For this review, take the finished solid that the model builds, in its own axes (mm). Face numbers are marked on the shaded views. Give positions to 0.01 mm unless a question says otherwise; leave off trailing zeros. Loops run counter-clockwise (first coordinate to the right, second up) from the corner with the lowest first, then second, coordinate; pieces in that order, holes last. Notation, with made-up numbers: (-17.5, 12) - (-2.5, 12) arc R11 ccw to (-2.5, 28) - close; hole circle Ø8 at (-3.75, -38). An arc over 180 degrees is marked (long way). Answer in a Markdown table with one row per item.
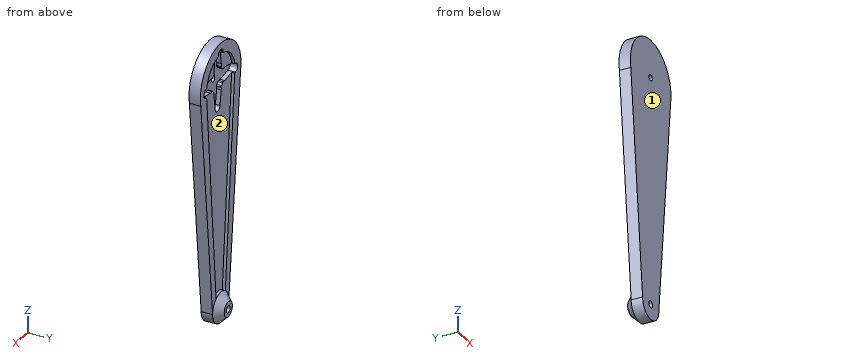
Autodesk Inventor part; units mm, degrees
ref_plane "Work Plane1" through (0, 12.5, 0) normal (0, 1, 0) x (1, 0, 0)
ref_plane "Work Plane2" through (0, 12.5, 0) normal (0, 1, 0) x (1, 0, 0)
ref_plane "YZ Plane" through (0, 0, 0) normal (1, 0, 0) x (0, 1, 0)
sketch "Sketch1" plane through (0, 0, 0) normal (0, 1, 0) x (-1, 0, 0)
  circle A0 centre (0, 0) radius 25
  line L0 (0, 0) -> (0, -150)
  circle A1 centre (0, -150) radius 10
  line L1 (0, 0) -> (25, 0)
  line L2 (0, -150) -> (10, -150)
  line L3 (0, -150) -> (-10, -150)
  line L4 (0, 0) -> (-25, 0)
  line L5 (25, 0) -> (10, -150)
  line L6 (-25, 0) -> (-10, -150)
  dimension "d0" = 50
  dimension "d1" = 150
  dimension "d2" = 20
extrude "Extrusion1" add sketch "Sketch1" along normal blind 7.5
sketch "Sketch2" plane through (0, 7.5, 0) normal (0, 1, 0) x (1, 0, 0)
  circle A0 centre (0, 0) radius 17.5
  arc A1 (10, 150) -> (-10, 150) centre (0, 150) ccw
  circle A2 centre (0, 150) radius 5
  line L0 (0, 0) -> (-17.5, 0)
  line L1 (0, 0) -> (17.5, 0)
  line L2 (0, 150) -> (-5, 150)
  line L3 (0, 150) -> (5, 150)
  line L4 (-17.5, 0) -> (-5, 150)
  line L5 (5, 150) -> (17.5, 0)
  dimension "d5" = 35
  dimension "d6" = 10
extrude "Extrusion2" cut sketch "Sketch2" against normal blind 2 contours L4 A0 L5 L1 L0 | L4 A2 L5 A0
sketch "Sketch3" plane through (0, 5.5, 0) normal (0, 1, 0) x (1, 0, 0)
  arc A0 (5, 150) -> (-5, 150) centre (0, 150) ccw
  circle A1 centre (0, 150) radius 2.25
  circle A2 centre (0, 0) radius 2
  dimension "d9" = 4.5
  dimension "d12" = 4
extrude "Extrusion4" cut sketch "Sketch3" against normal blind 5.5
sketch "Sketch4" plane through (0, 7.5, 0) normal (0, 1, 0) x (1, 0, 0)
  circle A0 centre (0, 150) radius 2.25
  arc A1 (5, 150) -> (-5, 150) centre (0, 150) ccw
  arc A2 (10, 150) -> (-10, 150) centre (0, 150) ccw
  line L0 (24.505, 4.9505) -> (10, 150)
  circle A3 centre (0, 150) radius 10
  circle A4 centre (0, 150) radius 2.25
  point P0 (0, 0)
  dimension "d22" = 4.5
ref_plane "Work Plane1" through (0, 12.5, 0) normal (0, 1, 0) x (1, 0, 0)
sketch "Sketch8" plane through (0, 5.5, 0) normal (0, 1, 0) x (1, 0, 0)
  point P0 (0, 0)
sketch "Sketch9" plane through (0, 7.5, 0) normal (0, 1, 0) x (1, 0, 0)
  arc A0 (2, 0) -> (-2, 0) centre (0, 0) ccw
  line L0 (17.5, 0) -> (-17.5, 0)
  circle A1 centre (0, 0) radius 17.5
extrude "Extrusion7" cut sketch "Sketch9" against normal blind 2 contours A0 L0 A1 | L0 A1
sketch "Sketch10" plane through (0, 7.5, 0) normal (0, 1, 0) x (1, 0, 0)
  arc A0 (-2.0881, -18.0545) -> (1.8643, -18.079) centre (-0.11, -17.7593) ccw
  line L0 (3.4056, -8.5599) -> (1.8643, -18.079)
  arc A1 (3.4056, -8.5599) -> (3.3448, -7.1465) centre (-0.0494, -8.0004) ccw
  arc A2 (4.0411, -5.092) -> (3.3448, -7.1465) centre (5.2844, -6.6585) ccw
  arc A3 (4.0411, -5.092) -> (5.0411, -4.1043) centre (0.0003, -0.0006) ccw
  arc A4 (7.1041, -3.4336) -> (5.0411, -4.1043) centre (6.5921, -5.367) ccw
  arc A5 (7.1041, -3.4336) -> (8.5166, -3.512) centre (8.0001, -0.0503) ccw
  line L1 (18.0541, -2.089) -> (8.5166, -3.512)
  arc A6 (18.0541, -2.089) -> (18.0787, 1.8634) centre (17.759, -0.1109) ccw
  line L2 (8.5596, 3.4047) -> (18.0787, 1.8634)
  arc A7 (8.5596, 3.4047) -> (7.1462, 3.344) centre (8.0001, -0.0503) ccw
  arc A8 (5.0917, 4.0402) -> (7.1462, 3.344) centre (6.6582, 5.2835) ccw
  arc A9 (5.0917, 4.0402) -> (4.104, 5.0402) centre (0.0003, -0.0006) ccw
  arc A10 (3.4333, 7.1032) -> (4.104, 5.0402) centre (5.3667, 6.5912) ccw
  arc A11 (3.4333, 7.1032) -> (3.5117, 8.5157) centre (0.05, 7.9993) ccw
  line L3 (2.0887, 18.0533) -> (3.5117, 8.5157)
  arc A12 (2.0887, 18.0533) -> (-1.8637, 18.0778) centre (0.1106, 17.7581) ccw
  line L4 (-3.405, 8.5587) -> (-1.8637, 18.0778)
  arc A13 (-3.405, 8.5587) -> (-3.3443, 7.1453) centre (0.05, 7.9993) ccw
  arc A14 (-4.0405, 5.0908) -> (-3.3443, 7.1453) centre (-5.2838, 6.6574) ccw
  arc A15 (-4.0405, 5.0908) -> (-5.0405, 4.1031) centre (0.0003, -0.0006) ccw
  arc A16 (-7.1035, 3.4325) -> (-5.0405, 4.1031) centre (-6.5915, 5.3658) ccw
  arc A17 (-7.1035, 3.4325) -> (-8.516, 3.5108) centre (-7.9996, 0.0491) ccw
  line L5 (-18.0536, 2.0878) -> (-8.516, 3.5108)
  arc A18 (-18.0536, 2.0878) -> (-18.0781, -1.8646) centre (-17.7585, 0.1097) ccw
  line L6 (-8.559, -3.4059) -> (-18.0781, -1.8646)
  arc A19 (-8.559, -3.4059) -> (-7.1456, -3.3451) centre (-7.9996, 0.0491) ccw
  arc A20 (-5.0911, -4.0414) -> (-7.1456, -3.3451) centre (-6.6577, -5.2847) ccw
  arc A21 (-5.0911, -4.0414) -> (-4.1034, -5.0414) centre (0.0003, -0.0006) ccw
  arc A22 (-3.4328, -7.1044) -> (-4.1034, -5.0414) centre (-5.3661, -6.5924) ccw
  arc A23 (-3.4328, -7.1044) -> (-3.5111, -8.5169) centre (-0.0494, -8.0004) ccw
  line L7 (-2.0881, -18.0545) -> (-3.5111, -8.5169)
  arc A24 (-18.2011, 3.0769) -> (-18.238, -2.8517) centre (-17.7585, 0.1097) ccw
  line L8 (-18.2011, 3.0769) -> (-8.6636, 4.4998)
  arc A25 (-6.8475, 4.3991) -> (-8.6636, 4.4998) centre (-7.9996, 0.0491) ccw
  arc A26 (-6.8475, 4.3991) -> (-5.816, 4.7345) centre (-6.5915, 5.3658) ccw
  arc A27 (-4.6622, 5.8741) -> (-5.816, 4.7345) centre (0.0003, -0.0006) ccw
  arc A28 (-4.6622, 5.8741) -> (-4.314, 6.9013) centre (-5.2838, 6.6574) ccw
  arc A29 (-4.3922, 8.7185) -> (-4.314, 6.9013) centre (0.05, 7.9993) ccw
  line L9 (-4.3922, 8.7185) -> (-2.8509, 18.2377)
  arc A30 (3.0777, 18.2008) -> (-2.8509, 18.2377) centre (0.1106, 17.7581) ccw
  line L10 (3.0777, 18.2008) -> (4.5007, 8.6633)
  arc A31 (4.4, 6.8472) -> (4.5007, 8.6633) centre (0.05, 7.9993) ccw
  arc A32 (4.4, 6.8472) -> (4.7353, 5.8157) centre (5.3667, 6.5912) ccw
  arc A33 (5.8749, 4.6619) -> (4.7353, 5.8157) centre (0.0003, -0.0006) ccw
  arc A34 (5.8749, 4.6619) -> (6.9022, 4.3137) centre (6.6582, 5.2835) ccw
  arc A35 (8.7194, 4.3919) -> (6.9022, 4.3137) centre (8.0001, -0.0503) ccw
  line L11 (8.7194, 4.3919) -> (18.2385, 2.8505)
  arc A36 (18.2017, -3.078) -> (18.2385, 2.8505) centre (17.759, -0.1109) ccw
  line L12 (18.2017, -3.078) -> (8.6642, -4.501)
  arc A37 (6.8481, -4.4003) -> (8.6642, -4.501) centre (8.0001, -0.0503) ccw
  arc A38 (6.8481, -4.4003) -> (5.8166, -4.7356) centre (6.5921, -5.367) ccw
  arc A39 (4.6627, -5.8753) -> (5.8166, -4.7356) centre (0.0003, -0.0006) ccw
  arc A40 (4.6627, -5.8753) -> (4.3146, -6.9025) centre (5.2844, -6.6585) ccw
  arc A41 (4.3927, -8.7197) -> (4.3146, -6.9025) centre (-0.0494, -8.0004) ccw
  line L13 (4.3927, -8.7197) -> (2.8514, -18.2388)
  arc A42 (-3.0772, -18.202) -> (2.8514, -18.2388) centre (-0.11, -17.7593) ccw
  line L14 (-3.0772, -18.202) -> (-4.5001, -8.6645)
  arc A43 (-4.3994, -6.8484) -> (-4.5001, -8.6645) centre (-0.0494, -8.0004) ccw
  arc A44 (-4.3994, -6.8484) -> (-4.7348, -5.8169) centre (-5.3661, -6.5924) ccw
  arc A45 (-5.8744, -4.663) -> (-4.7348, -5.8169) centre (0.0003, -0.0006) ccw
  arc A46 (-5.8744, -4.663) -> (-6.9016, -4.3149) centre (-6.6577, -5.2847) ccw
  arc A47 (-8.7188, -4.3931) -> (-6.9016, -4.3149) centre (-7.9996, 0.0491) ccw
  line L15 (-8.7188, -4.3931) -> (-18.238, -2.8517)
  point P0 (0, 0)
  point P1 (-0.0006, -0.0008)
  point P2 (5.0634, 6.1933)
  point P3 (0.0701, 8.4991)
  point P4 (0.0003, -0.0006)
  point P5 (11.2399, 13.7492)
  point P6 (5.0634, 6.1933)
  point P7 (6.1942, -5.0637)
  point P8 (13.7501, -11.2402)
  point P9 (-13.7495, 11.239)
  point P10 (-11.2393, -13.7504)
  point P11 (-5.0629, -6.1945)
  point P12 (-5.0629, -6.1945)
  point P13 (-0.0695, -8.5003)
  point P14 (0.0003, -0.0006)
  dimension "d38" = 0.001
  dimension "d39" = 1
extrude "Extrusion8" cut sketch "Sketch10" against normal blind 5 contours L7 A23 A22 A21 A20 A19 L6 A18 L5 A17 A16 A15 A14 A13 L4 A12 L3 A11 A10 A9 A8 A7 L2 A6 L1 A5 A4 A3 A2 A1 L0 A0 | L8 A25 A26 A27 A28 A29 L9 A30 L10 A31 A32 A33 A34 A35 L11 A36 L12 A37 A38 A39 A40 A41 L13 A42 L14 A43 A44 A45 A46 A47 L15 A24
extrude "Extrusion9" add sketch "Sketch4" against normal blind 5
sketch "Sketch11" plane through (0, 7.5, 0) normal (0, 1, 0) x (1, 0, 0)
  circle A0 centre (0, 150) radius 2.25
  line L0 (24.505, 4.9505) -> (10, 150)
  circle A1 centre (0, 150) radius 10
  point P0 (0, 0)
ref_plane "Work Plane2" through (0, 12.5, 0) normal (0, 1, 0) x (1, 0, 0)
sketch "Sketch12" plane through (0, 12.5, 0) normal (0, 1, 0) x (1, 0, 0)
  circle A0 centre (0, 150) radius 2.25
  circle A1 centre (0, 150) radius 5
  point P0 (0, 0)
  dimension "d45" = 10
loft "Loft3" add profiles "Sketch11", "Sketch12" contours A0 | A1 / A0 | A1
sketch "Sketch13" plane through (0, 12.5, -150) normal (0, 1, 0) x (1, 0, 0)
  circle A0 centre (0, 0) radius 2.25
  circle A1 centre (0, 0) radius 2.25
  point P0 (0, -150)
  dimension "d50" = 4.5
extrude "Extrusion10" cut sketch "Sketch13" against normal blind 10
properties part number "Delta_Arm"
1. We need section B-B, the plane y = 10.25. Give the boundary of the cut face in (x, z).
Values:
| item | result |
|---|---|
| outline | circle Ø14.5 at (0, -150); hole circle Ø4.5 at (0, -150) |
2. Wall thickness on line 1 (Z direction, x = 0, y = 1.3); line 2 (X direction, y = 0.75, z = 0); line 3 (X direction, y = 2.75, z = -150): over which ranges is each line inside the solid? List them lowest first. Write a range as [from, to].
Values:
| item | result |
|---|---|
| line 1 | z = [-160, -152.25], [-147.75, -2], [2, 25] |
| line 2 | x = [-25, -2], [2, 25] |
| line 3 | x = [-10, -2.25], [2.25, 10] |
3. Clearance check with flat-ended pins moving along their axes: pin 1 (5 mm diameter, centred on x = 5, z = -32.5, fed in from +Y); pin 2 (21 mm diameter, centred on x = 10, z = -9.5, fed in from +Y); pin 3 (2 mm diameter, centred on y = 4.5, z = -100, fed in from -X). State where each tip first meets the part, or that it passes through.
Values:
| item | result |
|---|---|
| pin 1 | stops at y = 5.5 |
| pin 2 | stops at y = 7.5 |
| pin 3 | stops at x = -15.1 |
4. We need section A-A, the plane x = 0. Give the boundary of the cut face in (y, z), and give its area (3 significant figures).
Values:
| item | result |
|---|---|
| outline | (0, -160) - (7.5, -160) - (12.5, -155) - (12.5, -152.25) - (0, -152.25) - close; (0, -147.75) - (12.5, -147.75) - (12.5, -145) - (7.5, -140) - (5.5, -140) - (5.5, -20.76) - (2.5, -20.76) - (2.5, -2) - (0, -2) - close; (0, 2) - (2.5, 2) - (2.5, 20.76) - (7.5, 20.76) - (7.5, 25) - (0, 25) - close |
| area | 950 mm^2 |
5. We need section C-C, the plane z = -95.5. Give the boundary of the cut face in (x, y).
Values:
| item | result |
|---|---|
| outline | (-15.45, 0) - (15.45, 0) - (15.45, 7.5) - (9.54, 7.5) - (9.54, 5.5) - (-9.54, 5.5) - (-9.54, 7.5) - (-15.45, 7.5) - close |
6. Mouldability with a two-part tool opening along X and no side actions: class the marked faces 1 and 2 as released by +X, released by -X, zero draft, split by the parting line, or undercut.
Values:
| item | result |
|---|---|
| face 1 | zero draft |
| face 2 | undercut |
7. We need section D-D, the plane z = -22.5. Give the boundary of the cut face in (x, y) (3 decimals).
Values:
| item | result |
|---|---|
| outline | (-22.75, 0) - (22.75, 0) - (22.75, 7.5) - (15.625, 7.5) - (15.625, 5.5) - (-15.625, 5.5) - (-15.625, 7.5) - (-22.75, 7.5) - close |
